Autodesk Inventor part; units mm, degrees
ref_plane "YZ Plane" through (0, 0, 0) normal (1, 0, 0) x (0, 1, 0)
ref_plane "XZ Plane" through (0, 0, 0) normal (0, 1, 0) x (-1, 0, 0)
ref_plane "XY Plane" through (0, 0, 0) normal (0, 0, 1) x (1, 0, 0)
ref_plane "Work Plane1" through (0, 0, 0) normal (0, 0, 1) x (1, 0, 0)
sketch "Sketch1" plane through (0, 0, 0) normal (0, 0, 1) x (1, 0, 0)
  line L0 (27.9999, -0.0002) -> (27.9999, 599.9998)
  line L1 (-2, -0.0002) -> (-2, 599.9998)
  line L2 (-75.0445, 277.7834) -> (27.9999, 277.7834)
  line L3 (27.9999, 277.7834) -> (27.9999, 322.2162)
  line L4 (27.9999, 322.2162) -> (-75.0445, 322.2162)
  line L5 (-75.0445, 322.2162) -> (-75.0445, 277.7834)
  line L6 (-75.0445, 277.7834) -> (27.9999, 322.2162) construction
  line L7 (27.9999, 277.7834) -> (-75.0445, 322.2162) construction
  line L8 (-5.6506, 302.4998) -> (-67.1503, 302.4998)
  line L9 (-66.9479, 297.5039) -> (-5.7013, 297.5039)
  line L10 (-5.6506, 302.4998) -> (-66.9479, 297.5039) construction
  line L11 (-67.1503, 302.4998) -> (-5.7013, 297.5039) construction
  arc A0 (-67.1503, 302.4998) -> (-66.9479, 297.5039) centre (-67.3544, 299.9894) ccw
  arc A1 (-5.7013, 297.5039) -> (-5.9109, 302.4785) centre (-5.578, 300.0008) ccw
  line L12 (27.9999, 277.7834) -> (12.9999, 277.7834)
  circle A2 centre (12.9999, 287.7834) radius 2.5
  circle A3 centre (12.9999, 312.2162) radius 2.5
  line L13 (12.9999, 277.7834) -> (12.9999, 285.2834)
  point P0 (0, 0)
  point P1 (-23.5223, 299.9998)
  point P2 (-36.3624, 299.9967)
  dimension "d4" = 5
  dimension "d0" = 5
  dimension "d1" = 15
  dimension "d5" = 5
extrude "Extrusion1" add sketch "Sketch1" along normal blind 6
fillet "Fillet1" radius 15 2 edges at (-75.0445, 277.7834, 3) (-75.0445, 322.2162, 3)
properties part number "Idler"
Here's how the part is built. I have some questions about the finished solid (model axes, mm). A direction names the side the tool comes from. Coordinates: 2 decimals unless noted, no trailing zeros. Order: outer loops, then holes, each group sorted by start corner. A loop starts at its lowest first (then second) coordinate and runs counter-clockwise, first axis right, second up. Notation, with made-up numbers: M -3,45 L 35,45 A17 ccw 35,61 Z; hole C 6.25,73.25 d7. An arc over 180 degrees is marked long. Answer as a JSON object with one key per item and string values. Group by question number.
(1) Suppose I cut it at C-C, the plane z = 4.1. Please give me the cut outline in (x, y).
(2) Suppose I cut it at A-A, the plane x = -8.5. Please give me the cut outline in (y, z), then the cut area to 3 significant figures.
(3) If we mould it in two halves opening along X, with no side actions, what happens to faces 3 (the face through (-3.08, 300.03, 2.96)), 4 (the face through (-75.044, 300, 3)), 5 (the face through (-37, 297.504, 3)), 6 (the face through (-24, 305, 6))? For each: released by +X, released by -X, zero draft, split by the parting line, or undercut.
(4) I need wall thicknesses on probe 1 along Y at (x, z) = (-10, 1.3); probe 2 along Y at (x, z) = (13.5, 2); probe 3 along Y at (x, z) = (12, 4.65). Which ranges of each line are inside material? Lowest first, please.
(5) Suppose I cut it at D-D, the plane y = 282. Please give me the cut outline in (x, z).
(6) Which directions (+Z, -Z, +X, -X, +Y, -Y) give clear straight access to the entire face, cutting with the end or side of a thin tool? Please do faces 1 (the face through (-70.53, 317.94, 3.04)), 2 (the face through (-36, 302.5, 3)).
(7) Suppose I cut it at B-B, the plane y = 301. Please give me the cut outline in (x, z), then the cut area to 3 significant figures.
Values found:
{
 "1": {"outline": "M -75.04,292.78 A15 ccw -60.04,277.78 L 28,277.78 L 28,322.22 L -60.04,322.22 A15 ccw -75.04,307.22 Z; hole M -67.15,302.5 A2.52 ccw long -66.95,297.5 L -5.7,297.5 A2.5 ccw long -5.65,302.5 Z; hole C 13,287.78 d5; hole C 13,312.22 d5"},
 "2": {"outline": "M 277.78,0 L 297.5,0 L 297.5,6 L 277.78,6 Z; M 302.5,0 L 322.22,0 L 322.22,6 L 302.5,6 Z", "area": "237 mm^2"},
 "3": {"face 3": "undercut", "face 4": "released by -X", "face 5": "undercut", "face 6": "zero draft"},
 "4": {"probe 1": "y = 277.78 to 297.5, 302.5 to 322.22", "probe 2": "y = 277.78 to 285.33, 290.23 to 309.77, 314.67 to 322.22", "probe 3": "y = 277.78 to 285.49, 290.07 to 309.92, 314.51 to 322.22"},
 "5": {"outline": "M -70.47,0 L 28,0 L 28,6 L -70.47,6 Z"},
 "6": {"face 1": "+Z, -Z, -X, +Y", "face 2": "+Z, -Z"},
 "7": {"outline": "M -75.04,0 L -69.66,0 L -69.66,6 L -75.04,6 Z; M -3.29,0 L 28,0 L 28,6 L -3.29,6 Z", "area": "220 mm^2"}
}
